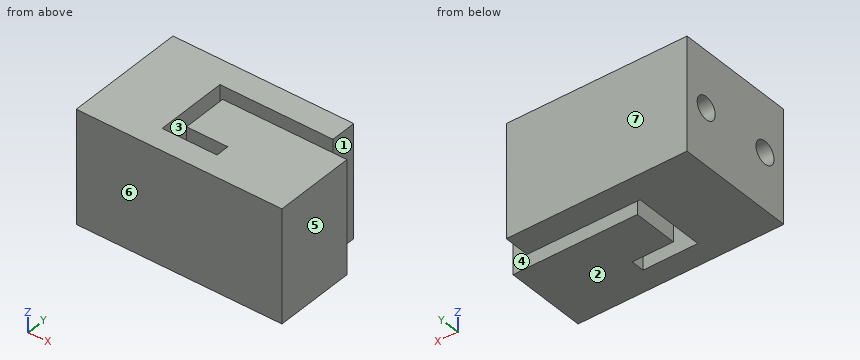
Autodesk Inventor part; units mm, degrees
ref_plane "YZ Plane" through (0, 0, 0) normal (1, 0, 0) x (0, 1, 0)
ref_plane "XZ Plane" through (0, 0, 0) normal (0, 1, 0) x (-1, 0, 0)
ref_plane "XY Plane" through (0, 0, 0) normal (0, 0, 1) x (1, 0, 0)
sketch "Sketch1" plane through (0, 0, 0) normal (0, 0, 1) x (1, 0, 0)
  line L0 (0, 7.7) -> (0, 1.3)
  line L1 (1.2, 6.5) -> (12.2, 6.5)
  line L2 (1.2, 2.5) -> (4.8537, 2.5)
  line L3 (1.2, 6.5) -> (1.2, 2.5)
  line L4 (0, 1.3) -> (4.8537, 1.3)
  line L5 (4.8537, 2.5) -> (4.8537, 1.3)
  line L6 (12.2, -0.7) -> (12.2, 6.5)
  line L7 (0, 7.7) -> (10, 7.7)
  line L8 (10, 7.7) -> (10, 10)
  line L9 (-6, 10) -> (-6, -0.7)
  line L10 (-6, 10) -> (10, 10)
  line L11 (-6, -0.7) -> (12.2, -0.7)
  dimension "d7" = 1.2
  dimension "d9" = 1.2
  dimension "d10" = 11
  dimension "d12" = 1.2
  dimension "d13" = 4
  dimension "d21" = 6
extrude "Extrusion3" add sketch "Sketch1" along normal blind 10
sketch "Sketch3" plane through (-6, -0.7, 0) normal (-1, 0, 0) x (0, 0, 1)
  circle A0 centre (5, 8.5811) radius 1
  circle A1 centre (5, 2.0811) radius 1
  line L0 (0, 0) -> (0, 10.7)
  line L1 (0, 0) -> (10, 0)
  line L2 (10, 10.7) -> (10, 0)
  line L3 (0, 10.7) -> (10, 10.7)
  line L4 (5, 10.7) -> (5, 0)
  point P0 (0, 0.7)
  dimension "d24" = 2
  dimension "d25" = 2
  dimension "d26" = 6.5
extrude "Extrusion4" cut sketch "Sketch3" against normal blind 6 contours A0 L4 | L4 A0 | L4 A1 | A1 L4
properties part number "endstop mount"
Input: part model. Units: mm. Frame: model coordinates. Face numbers are marked on the shaded views. A direction names the side the tool comes from. Give positions to 0.01 mm unless a question says otherwise; leave off trailing zeros. Write each loop counter-clockwise with the first axis right and the second up, starting at its lowest first coordinate (ties: lowest second). Pieces come first, ordered by that corner, then holes.
Q1. Set-up query: the marked faces 1, 2 and 3. Return all of +Z, -Z, +X, -X, +Y, -Y with unobstructed straight access to the full face (end or side cutting, diameter ignored); none if empty.
Q2. Section D-D, the plane z = 9. Output: boundary loops of the cut face in (x, y), plus the area to 3 significant figures.
Q3. Section B-B, the plane y = 4.5. Output: boundary loops of the cut face in (x, z), plus the area to 3 significant figures.
Q4. Material intervals for probe 1 along Y at (x, z) = (-2.85, 5); probe 2 along X at (y, z) = (4, 2.25); probe 3 along X at (y, z) = (2.25, 3.75), sorted ascending.
Q5. First-contact query: P1, Ø2.5, axis at y = 7.88, z = 5, coming from the +X side. Flat tip, straight axial feed; report the tip coordinate or a pass-through.
Q6. Pull-direction query (Y, two-part tool) for the marked faces 4, 5, 6 and 7; classes: pulls with the +Y half, pulls with the -Y half, needs draft (parallel to the pull), parting line crosses it, or undercut.
Q7. Section A-A, the plane z = 5. Output: boundary loops of the cut face in (x, y).
Q8. Section C-C, the plane x = 1. Output: boundary loops of the cut face in (y, z).
Filled in:
1. face 1: +Z, -Z, +X, +Y
1. face 2: -Z, +X, -X, +Y, -Y
1. face 3: +Z, -Z
2. outline: (-6, -0.7) - (12.2, -0.7) - (12.2, 6.5) - (1.2, 6.5) - (1.2, 2.5) - (4.85, 2.5) - (4.85, 1.3) - (0, 1.3) - (0, 7.7) - (10, 7.7) - (10, 10) - (-6, 10) - close
2. area: 164 mm2
3. outline: (-6, 0) - (0, 0) - (0, 10) - (-6, 10) - close; (1.2, 0) - (12.2, 0) - (12.2, 10) - (1.2, 10) - close
3. area: 170 mm2
4. probe 1: y = -0.7 to 0.38, 2.38 to 6.88, 8.88 to 10
4. probe 2: x = -6 to 0, 1.2 to 12.2
4. probe 3: x = -6 to 0, 4.85 to 12.2
5. P1: stops at x = 10
6. face 4: undercut
6. face 5: needs draft
6. face 6: pulls with the -Y half
6. face 7: pulls with the +Y half
7. outline: (-6, -0.7) - (12.2, -0.7) - (12.2, 6.5) - (1.2, 6.5) - (1.2, 2.5) - (4.85, 2.5) - (4.85, 1.3) - (0, 1.3) - (0, 0.38) - (-6, 0.38) - close; (-6, 2.38) - (0, 2.38) - (0, 6.88) - (-6, 6.88) - close; (-6, 8.88) - (0, 8.88) - (0, 7.7) - (10, 7.7) - (10, 10) - (-6, 10) - close
8. outline: (-0.7, 0) - (1.3, 0) - (1.3, 10) - (-0.7, 10) - close; (7.7, 0) - (10, 0) - (10, 10) - (7.7, 10) - close
